Could you check a few things on this model? Use its own coordinates, in mm. Coordinates: 2 decimals unless noted, no trailing zeros. Write each loop counter-clockwise with the first axis right and the second up, starting at its lowest first coordinate (ties: lowest second). Pieces come first, ordered by that corner, then holes. Notation, with made-up numbers: (8.25, 5.5) - (54.25, 5.5) arc R21 ccw to (54.25, 33.5) - close; hole circle Ø10 at (40.25, 35.5). An arc over 180 degrees is marked (long way). Answer as a JSON object with one key per item and string values. Group by question number.
1) Will these pins go through, and if not, where does the flat tip stop? pin 1 Ø2.5 at (y, z) = (-173.5, 3.5) entering from +X; pin 2 Ø3 at (y, z) = (22, 1) entering from -X; pin 3 Ø1.5 at (x, z) = (-241.5, 1.5) entering from -Y.
2) If we section it at D-D (y = -72.5): Write out the boundary of the cut face in (x, z), plus the area to 3 significant figures.
3) Please list where these lines run through material, in increasing order: line 1 along Y through (x, z) = (105.5, 2.7); line 2 along X through (y, z) = (107, 2.35); line 3 along Y through (x, z) = (-76, 2.35).
4) If we section it at A-A (y = 88): Write out the boundary of the cut face in (x, z), plus the area to 3 significant figures.
5) We'd pull the mould along X, two halves only. Please class faces 1 (the flat face through (-138, -66, 5)), 2 (the cylindrical face through (-107.66, -109.04, 2.46)): released by +X, released by -X, zero draft, split by the parting line, or undercut.
6) If we section it at B-B (x = -195): Write out the boundary of the cut face in (y, z), plus the area to 3 significant figures.
7) If we section it at C-C (x = -66): Write out the boundary of the cut face in (y, z), plus the area to 3 significant figures.
```python
from build123d import *

# Parameters (mm, degrees)
ESQUISSE1_W        = 5
ESQUISSE1_H        = 40
ESQUISSE1_W_2      = 40
ESQUISSE1_H_2      = 5
ESQUISSE1_W_3      = 80
ESQUISSE1_R        = 75
BOSS_EXTRU_1_DEPTH = 5


with BuildPart() as part:
    # Esquisse1 → Boss.-Extru.1 (new body)
    with BuildSketch(Plane.XY):
        Polygon((-238.142492866, -253.406593407), (-238.142492866, -263.406593407), (-228.142492866, -263.406593407), (-228.142492866, -258.406593407), (-208.142492866, -258.406593407), (-208.142492866, -263.406593407), (-168.142492866, -263.406593407), (-168.142492866, -258.406593407), (-88.142492866, -258.406593407), (-88.142492866, -263.406593407), (-8.142492866, -263.406593407), (-8.142492866, -258.406593407), (71.857507134, -258.406593407), (71.857507134, -263.406593407), (111.857507134, -263.406593407), (111.857507134, -258.406593407), (131.857507134, -258.406593407), (131.857507134, -263.406593407), (141.857507134, -263.406593407), (141.857507134, -253.406593407), (146.857507134, -253.406593407), (146.857507134, -213.406593407), (141.857507134, -213.406593407), (141.857507134, -93.406593407), (146.857507134, -93.406593407), (146.857507134, -53.406593407), (141.857507134, -53.406593407), (141.857507134, 76.593406593), (146.857507134, 76.593406593), (146.857507134, 116.593406593), (141.857507134, 116.593406593), (141.857507134, 126.593406593), (131.857507134, 126.593406593), (131.857507134, 121.593406593), (111.857507134, 121.593406593), (111.857507134, 126.593406593), (71.857507134, 126.593406593), (71.857507134, 121.593406593), (-8.142492866, 121.593406593), (-8.142492866, 126.593406593), (-88.142492866, 126.593406593), (-88.142492866, 121.593406593), (-168.142492866, 121.593406593), (-168.142492866, 126.593406593), (-208.142492866, 126.593406593), (-208.142492866, 121.593406593), (-228.142492866, 121.593406593), (-228.142492866, 126.593406593), (-238.142492866, 126.593406593), (-238.142492866, 116.593406593), (-243.142492866, 116.593406593), (-243.142492866, 76.593406593), (-238.142492866, 76.593406593), (-238.142492866, -53.406593407), (-243.142492866, -53.406593407), (-243.142492866, -93.406593407), (-238.142492866, -93.406593407), (-238.142492866, -213.406593407), (-243.142492866, -213.406593407), (-243.142492866, -253.406593407), align=None)
        with Locations((134.357507134, -233.406593407)):
            Rectangle(ESQUISSE1_W, ESQUISSE1_H, mode=Mode.SUBTRACT)
        with Locations((134.357507134, -73.406593407)):
            Rectangle(ESQUISSE1_W, ESQUISSE1_H, mode=Mode.SUBTRACT)
        with Locations((134.357507134, 96.593406593)):
            Rectangle(ESQUISSE1_W, ESQUISSE1_H, mode=Mode.SUBTRACT)
        with Locations((91.857507134, 114.093406593)):
            Rectangle(ESQUISSE1_W_2, ESQUISSE1_H_2, mode=Mode.SUBTRACT)
        with Locations((-48.142492866, 114.093406593)):
            Rectangle(ESQUISSE1_W_3, ESQUISSE1_H_2, mode=Mode.SUBTRACT)
        with Locations((-188.142492866, 114.093406593)):
            Rectangle(ESQUISSE1_W_2, ESQUISSE1_H_2, mode=Mode.SUBTRACT)
        with Locations((-230.642492866, 96.593406593)):
            Rectangle(ESQUISSE1_W, ESQUISSE1_H, mode=Mode.SUBTRACT)
        with Locations((-230.642492866, -73.406593407)):
            Rectangle(ESQUISSE1_W, ESQUISSE1_H, mode=Mode.SUBTRACT)
        with Locations((-230.642492866, -233.406593407)):
            Rectangle(ESQUISSE1_W, ESQUISSE1_H, mode=Mode.SUBTRACT)
        with Locations((-188.142492866, -250.906593407)):
            Rectangle(ESQUISSE1_W_2, ESQUISSE1_H_2, mode=Mode.SUBTRACT)
        with Locations((-48.142492866, -250.906593407)):
            Rectangle(ESQUISSE1_W_3, ESQUISSE1_H_2, mode=Mode.SUBTRACT)
        with Locations((91.857507134, -250.906593407)):
            Rectangle(ESQUISSE1_W_2, ESQUISSE1_H_2, mode=Mode.SUBTRACT)
        with Locations((-48.142492866, -63.406593407)):
            Circle(ESQUISSE1_R, mode=Mode.SUBTRACT)
    extrude(amount=BOSS_EXTRU_1_DEPTH)


solid = part.part
```
Here are the results:
{
 "1": {"pin 1": "stops at x = 141.86", "pin 2": "stops at x = -238.14", "pin 3": "stops at y = -253.41"},
 "2": {"outline": "(-243.14, 0) - (-233.14, 0) - (-233.14, 5) - (-243.14, 5) - close; (-228.14, 0) - (-122.59, 0) - (-122.59, 5) - (-228.14, 5) - close; (26.3, 0) - (131.86, 0) - (131.86, 5) - (26.3, 5) - close; (136.86, 0) - (146.86, 0) - (146.86, 5) - (136.86, 5) - close", "area": "1,160 mm²"},
 "3": {"line 1": "y = -263.41 to -253.41, -248.41 to 111.59, 116.59 to 126.59", "line 2": "x = -243.14 to -233.14, -228.14 to 131.86, 136.86 to 146.86", "line 3": "y = -263.41 to -253.41, -248.41 to -133.04, 6.23 to 111.59, 116.59 to 126.59"},
 "4": {"outline": "(-243.14, 0) - (-233.14, 0) - (-233.14, 5) - (-243.14, 5) - close; (-228.14, 0) - (131.86, 0) - (131.86, 5) - (-228.14, 5) - close; (136.86, 0) - (146.86, 0) - (146.86, 5) - (136.86, 5) - close", "area": "1,900 mm²"},
 "5": {"face 1": "zero draft", "face 2": "undercut"},
 "6": {"outline": "(-263.41, 0) - (-253.41, 0) - (-253.41, 5) - (-263.41, 5) - close; (-248.41, 0) - (111.59, 0) - (111.59, 5) - (-248.41, 5) - close; (116.59, 0) - (126.59, 0) - (126.59, 5) - (116.59, 5) - close", "area": "1,900 mm²"},
 "7": {"outline": "(-263.41, 0) - (-253.41, 0) - (-253.41, 5) - (-263.41, 5) - close; (-248.41, 0) - (-136.25, 0) - (-136.25, 5) - (-248.41, 5) - close; (9.44, 0) - (111.59, 0) - (111.59, 5) - (9.44, 5) - close; (116.59, 0) - (126.59, 0) - (126.59, 5) - (116.59, 5) - close", "area": "1,170 mm²"}
}
